Read the model definition and answer for the solid it produces. Units are mm, in the model's axes. A direction names the side the tool comes from. Coordinates: 2 decimals unless noted, no trailing zeros. Loops run counter-clockwise (first coordinate to the right, second up) from the corner with the lowest first, then second, coordinate; pieces in that order, holes last. Notation, with made-up numbers: (-1, 85.5) - (46, 85.5) arc R20 cw to (46, 109.5) - close; hole circle Ø8 at (-37.5, 2). An arc over 180 degrees is marked (long way). Use one line per item in the form item = value. Start each with the question number.
1) Each of these flat-tipped pins is pushed along its axis until it touches: P1, Ø12, axis at y = -9.5, z = -30, coming from the -X side; P2, Ø16, axis at y = 0, z = -35, coming from the +X side. Where does it stop, or does it pass through?
2) Which of the six approach directions +Z, -Z, +X, -X, +Y, -Y give full straight-line access (tool end or side, diameter ignored) to faces 4 (the face through (7, 25, -25)), 5 (the face through (25.289, -26.196, -24.72))?
3) The mould has two halves that part along Z. Classify faces 1 (the face through (25, 4, -5)), 2 (the face through (6, 28, -25)), 3 (the face through (26, 0, -30)): released by +Z, released by -Z, zero draft, split by the parting line, or undercut.
4) A cutting plane is placed at B-B (x = 7). Give the vertices of the cut face in (y, z).
5) A cutting plane is placed at C-C (y = 0). Give the vertices of the cut face in (x, z).
6) A cutting plane is placed at D-D (z = -15). Give the vertices of the cut face in (x, y).
7) Consider line 1 (Y direction, x = 6, z = -29); line 2 (X direction, y = -15, z = -17); line 3 (Y direction, x = 26.15, z = -35). Determine where each line is inside the solid, lowest interval first.
8) A cutting plane is placed at A-A (z = -31). Give the vertices of the cut face in (x, y), and give its area (3 significant figures).
from build123d import *

# Parameters (mm, degrees)
BASE_FLANGE1_DEPTH = 50
SKETCH10_R         = 5
CUT_EXTRUDE2_DEPTH = 68.149087857
FILLET1_R          = 3
SKETCH11_W         = 62.490132504
SKETCH11_H         = 65.671220534
CUT_EXTRUDE4_DEPTH = 5


# Sheet-metal steps are written as plain solids
with BuildPart() as part:
    # Sketch3 → Base-Flange1 (new body)
    with BuildSketch(Plane.XY):
        with BuildLine():
            Line((-8, -25), (21, -25))
            ThreePointArc((21, -25), (23.121320344, -24.121320344), (24, -22))
            Line((24, -22), (24, 22))
            ThreePointArc((24, 22), (23.121320344, 24.121320344), (21, 25))
            Line((21, 25), (-8, 25))
            Line((-8, 25), (-8, 28))
            Line((-8, 28), (21, 28))
            ThreePointArc((21, 28), (25.242640687, 26.242640687), (27, 22))
            Line((27, 22), (27, -22))
            ThreePointArc((27, -22), (25.242640687, -26.242640687), (21, -28))
            Line((21, -28), (-8, -28))
            Line((-8, -28), (-8, -25))
        make_face()
    extrude(amount=-BASE_FLANGE1_DEPTH)

    # Sketch10 → Cut-Extrude2 (cut, through all)
    with BuildSketch(Plane(origin=(27, 0, 0), x_dir=(0, 0, -1), z_dir=(1, 0, 0))):
        with Locations((15, 0)):
            Circle(SKETCH10_R)
        with Locations((35, 0)):
            Circle(SKETCH10_R)
    extrude(amount=-CUT_EXTRUDE2_DEPTH, mode=Mode.SUBTRACT)

    # Fillet1
    fillet1_edges = [part.edges().sort_by_distance(p)[0] for p in [
        (-8, 26.5, 0),
        (-8, -26.5, 0),
        (-8, 26.5, -50),
        (-8, -26.5, -50),
    ]]
    fillet(fillet1_edges, radius=FILLET1_R)

    # Sketch11 → Cut-Extrude4 (cut)
    with BuildSketch(Plane.XY):
        Rectangle(SKETCH11_W, SKETCH11_H)
    cut_extrude4 = extrude(amount=-CUT_EXTRUDE4_DEPTH, mode=Mode.SUBTRACT)

    # Mirror1: Cut-Extrude4 across plane
    add(cut_extrude4.mirror(Plane.XY.offset(-25)), mode=Mode.SUBTRACT)


solid = part.part
Found:
q1.P1 = 24
q1.P2 = 27
q2.face_4 = +Z, -Z, -X
q2.face_5 = +Z, -Z, +X, -Y
q3.face_1 = released by +Z
q3.face_2 = zero draft
q3.face_3 = undercut
q4.outline = (-28, -45) - (-25, -45) - (-25, -5) - (-28, -5) - close; (25, -45) - (28, -45) - (28, -5) - (25, -5) - close
q5.outline = (24, -45) - (27, -45) - (27, -40) - (24, -40) - close; (24, -30) - (27, -30) - (27, -20) - (24, -20) - close; (24, -10) - (27, -10) - (27, -5) - (24, -5) - close
q6.outline = (-8, -28) - (21, -28) arc R6 ccw to (27, -22) - (27, -5) - (24, -5) - (24, -22) arc R3 cw to (21, -25) - (-8, -25) - close; (-8, 25) - (21, 25) arc R3 cw to (24, 22) - (24, 5) - (27, 5) - (27, 22) arc R6 ccw to (21, 28) - (-8, 28) - close
q7.line_1 = -28 to -25, 25 to 28
q7.line_2 = 24 to 27
q7.line_3 = -25.08 to -5, 5 to 25.08
q8.outline = (-8, -28) - (21, -28) arc R6 ccw to (27, -22) - (27, -3) - (24, -3) - (24, -22) arc R3 cw to (21, -25) - (-8, -25) - close; (-8, 25) - (21, 25) arc R3 cw to (24, 22) - (24, 3) - (27, 3) - (27, 22) arc R6 ccw to (21, 28) - (-8, 28) - close
q8.area = 330 mm^2
